Geometry: final body of the model. Coordinates: model frame, mm. Round coordinates to 2 decimals unless told otherwise and drop trailing zeros. Loops run counter-clockwise (first coordinate to the right, second up) from the corner with the lowest first, then second, coordinate; pieces in that order, holes last. Notation, with made-up numbers: (57.25, 53) - (104.25, 53) arc R30 cw to (104.25, 90) - close; hole circle Ø7 at (11, -8). An arc over 180 degrees is marked (long way). Write item = value, one per line. Start each with the question number.
Item 1: Section A-A (y = -3.25). Return loops of the section in (x, z) (1 decimal), plus the area to 3 significant figures.
Item 2: Section B-B (x = 37.5). Return loops of the section in (y, z) (3 decimals), plus the area to 3 significant figures.
Item 3: Line query: line 1 (Z direction, x = 12.5, y = -2.5) (3 decimals); line 2 (Y direction, x = 70, z = 2). Output: solid intervals per line, ascending. Write a range as from..to.
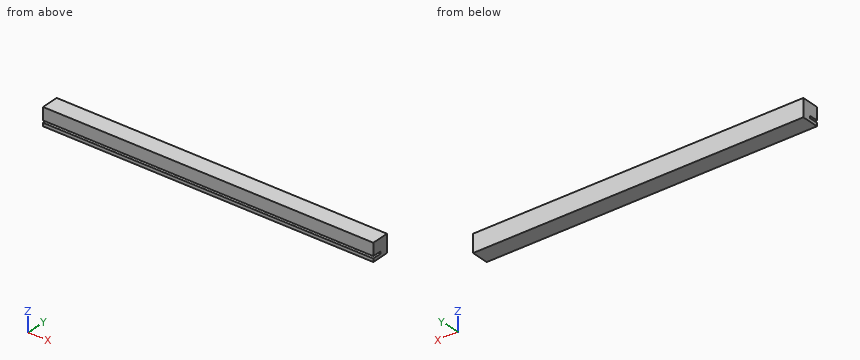
from build123d import *

# Parameters (mm, degrees)
SKETCH1_W           = 193.675
SKETCH1_H           = 10.16
BOSS_EXTRUDE1_DEPTH = 5.08
SKETCH2_W           = 193.675
SKETCH2_H           = 1.27
CUT_EXTRUDE1_DEPTH  = 5.334
SKETCH3_W           = 193.675
SKETCH3_H           = 10.16
BOSS_EXTRUDE2_DEPTH = 5.334


with BuildPart() as part:
    # Sketch1 → Boss-Extrude1 (new body)
    with BuildSketch(Plane.XY):
        Rectangle(SKETCH1_W, SKETCH1_H)
    extrude(amount=BOSS_EXTRUDE1_DEPTH)

    # Sketch2 → Cut-Extrude1 (cut)
    with BuildSketch(Plane.XZ.offset(5.08)):
        with Locations((0, 2.54)):
            Rectangle(SKETCH2_W, SKETCH2_H)
    extrude(amount=-CUT_EXTRUDE1_DEPTH, mode=Mode.SUBTRACT)

    # Sketch3 → Boss-Extrude2 (add)
    with BuildSketch(Plane.XY.offset(5.08)):
        Rectangle(SKETCH3_W, SKETCH3_H)
    extrude(amount=BOSS_EXTRUDE2_DEPTH)


solid = part.part
Taken from the geometry:
q1.outline = (-96.8, 0) - (96.8, 0) - (96.8, 1.9) - (-96.8, 1.9) - close; (-96.8, 3.2) - (96.8, 3.2) - (96.8, 10.4) - (-96.8, 10.4) - close
q1.area = 1,770 mm^2
q2.outline = (-5.08, 0) - (5.08, 0) - (5.08, 10.414) - (-5.08, 10.414) - (-5.08, 3.175) - (0.254, 3.175) - (0.254, 1.905) - (-5.08, 1.905) - close
q2.area = 99.0 mm^2
q3.line_1 = 0..1.905, 3.175..10.414
q3.line_2 = 0.25..5.08
